Geometry check sheet. Reference: drawing and pictorial views, mm from the part's lowest x, y, z. A direction names the side the tool comes from. Round coordinates to 2 decimals unless told otherwise and drop trailing zeros. Write each loop counter-clockwise with the first axis right and the second up, starting at its lowest first coordinate (ties: lowest second). Pieces come first, ordered by that corner, then holes. Notation, with made-up numbers: M 41.5,39.5 L 63.5,39.5 A21 ccw 63.5,46.5 Z; hole C 42.25,-37.75 d7. An arc over 180 degrees is marked long. Answer in a Markdown table with one row per item.
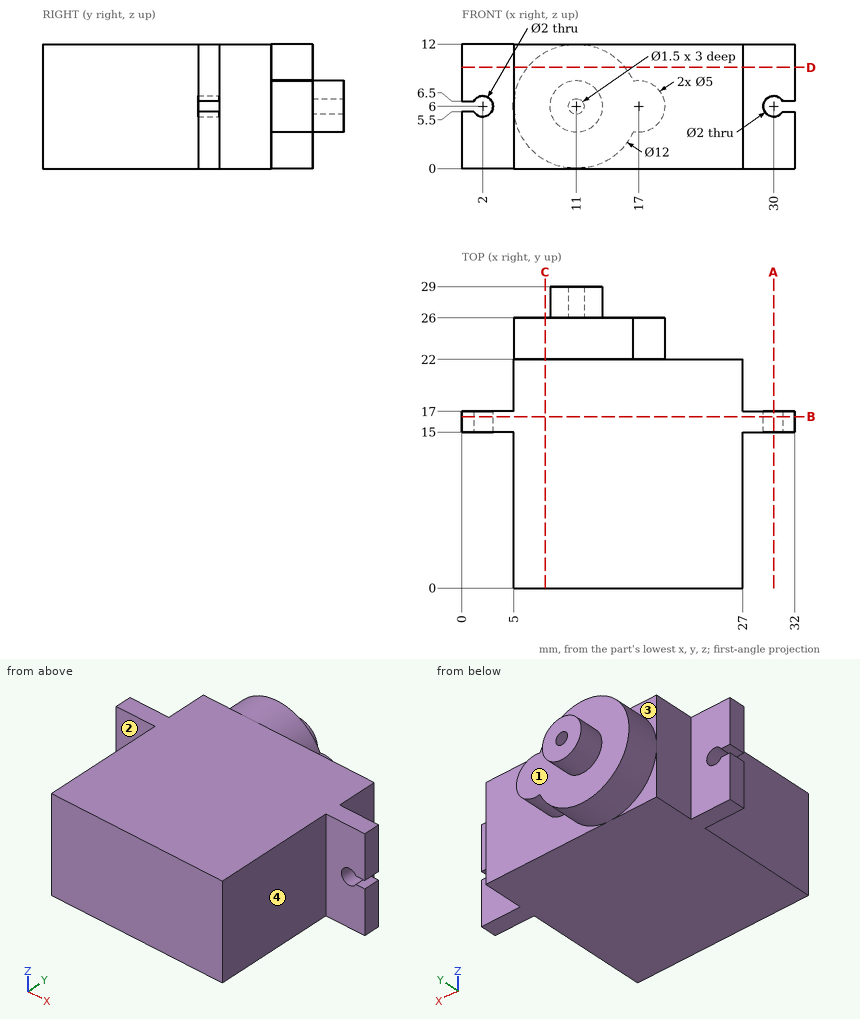
1. Section check A-A, the plane x = 30. Record the cut outline in (y, z).
Found:
| item | result |
|---|---|
| outline | M 15,0 L 17,0 L 17,5 L 15,5 Z; M 15,7 L 17,7 L 17,12 L 15,12 Z |
2. Scan lines: L1, parallel to X at y = 27.15, z = 6; L2, parallel to Y at x = 13.5, z = 10.75; L3, parallel to X at y = 7, z = 8.75. Record each from-to range of solid material in increasing order.
Found:
| item | result |
|---|---|
| L1 | x = 8.5 to 10.25, 11.75 to 13.5 |
| L2 | y = 0 to 26 |
| L3 | x = 5 to 27 |
3. Section check B-B, the plane y = 16.5. Record the cut outline in (x, z), and give its area (3 significant figures).
Found:
| item | result |
|---|---|
| outline | M 0,0 L 32,0 L 32,5.5 L 30.87,5.5 A1 cw long 30.87,6.5 L 32,6.5 L 32,12 L 0,12 L 0,6.5 L 1.13,6.5 A1 cw long 1.13,5.5 L 0,5.5 Z |
| area | 376 mm2 |
4. Access from +Z, -Z, +X, -X, +Y, -Y to the whole of each face (thin tool, end or side, straight path). Record for the marked faces 1, 2, 3 and 4.
Found:
| item | result |
|---|---|
| face 1 | +Y |
| face 2 | +Z, -Z, -X, -Y |
| face 3 | +Z, -X, +Y |
| face 4 | +Z, -Z, +X, -Y |
5. Go/stop test with flat-tipped pins: pin 1 (1.2 mm diameter, centred on x = 30, z = 6, fed in from -Y); pin 2 (3 mm diameter, centred on x = 19.5, z = 3.5, fed in from -Y); pin 3 (6 mm diameter, centred on y = 6, z = 8, fed in from +X); pin 4 (1.5 mm diameter, centred on x = 21, z = 6.5, fed in from +Y). Record where each tip stops, or that it passes through.
Found:
| item | result |
|---|---|
| pin 1 | passes through |
| pin 2 | stops at y = 0 |
| pin 3 | stops at x = 27 |
| pin 4 | stops at y = 22 |
6. Section check D-D, the plane z = 9.75. Record the cut outline in (x, y), and give its area (3 significant figures).
Found:
| item | result |
|---|---|
| outline | M 0,15 L 5,15 L 5,0 L 27,0 L 27,15 L 32,15 L 32,17 L 27,17 L 27,22 L 15.68,22 L 15.68,26 L 6.32,26 L 6.32,22 L 5,22 L 5,17 L 0,17 Z |
| area | 541 mm2 |
7. Section check C-C, the plane x = 8. Record the cut outline in (y, z).
Found:
| item | result |
|---|---|
| outline | M 0,0 L 22,0 L 22,0.8 L 26,0.8 L 26,11.2 L 22,11.2 L 22,12 L 0,12 Z |
